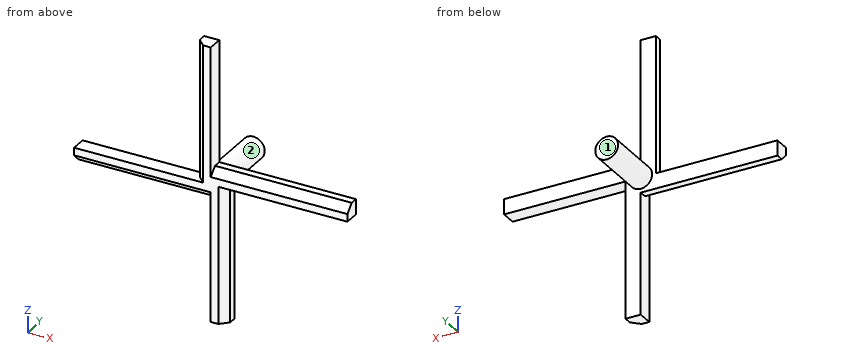
from build123d import *

# Parameters (mm, degrees)
F1_DEPTH = 10
F2_SIZE  = 5
F3_R     = 7.5
F4_DEPTH = 40


with BuildPart() as f1:
    # F0 (on Front) → F1 (new body)
    with BuildSketch(Plane.XZ):
        with BuildLine():
            ThreePointArc((-10, 0), (-7.0710678119, 7.0710678119), (0, 10))
            Line((0, 10), (0, 90))
            Line((0, 90), (-10, 90))
            Line((-10, 90), (-10, 0))
        make_face()
        with BuildLine():
            ThreePointArc((0, -10), (-7.0710678119, -7.0710678119), (-10, 0))
            Line((-10, 0), (-90, 0))
            Line((-90, 0), (-90, -10))
            Line((-90, -10), (0, -10))
        make_face()
        with BuildLine():
            Line((10, -90), (10, 0))
            ThreePointArc((10, 0), (7.0710678119, -7.0710678119), (0, -10))
            Line((0, -10), (0, -90))
            Line((0, -90), (10, -90))
        make_face()
        with BuildLine():
            Line((0, 10), (0, 0))
            Line((0, 0), (10, 0))
            ThreePointArc((10, 0), (7.0710678119, 7.0710678119), (0, 10))
        make_face()
        with BuildLine():
            Line((10, 0), (0, 0))
            Line((0, 0), (0, -10))
            ThreePointArc((0, -10), (7.0710678119, -7.0710678119), (10, 0))
        make_face()
        with BuildLine():
            Line((-10, 0), (0, 0))
            Line((0, 0), (0, 10))
            ThreePointArc((0, 10), (-7.0710678119, 7.0710678119), (-10, 0))
        make_face()
        with BuildLine():
            Line((0, -10), (0, 0))
            Line((0, 0), (-10, 0))
            ThreePointArc((-10, 0), (-7.0710678119, -7.0710678119), (0, -10))
        make_face()
        with BuildLine():
            ThreePointArc((0, 10), (7.0710678119, 7.0710678119), (10, 0))
            Line((10, 0), (90, 0))
            Line((90, 0), (90, 10))
            Line((90, 10), (0, 10))
        make_face()
    extrude(amount=F1_DEPTH)

    # F2
    f2_edges = [f1.edges().sort_by_distance(p)[0] for p in [
        (-10, -10, 45),
        (-45, -10, -10),
        (10, -10, -45),
        (45, -10, 10),
    ]]
    chamfer(f2_edges, length=F2_SIZE)

    # F3 (on Front) → F4 (join)
    with BuildSketch(Plane.XZ):
        Circle(F3_R)
    extrude(amount=-F4_DEPTH)


solid = f1.part
Geometry: final body of the model. Coordinates: model frame, mm. Face numbers are marked on the shaded views. A direction names the side the tool comes from. Give positions to 0.01 mm unless a question says otherwise; leave off trailing zeros. Loops run counter-clockwise (first coordinate to the right, second up) from the corner with the lowest first, then second, coordinate; pieces in that order, holes last. Notation, with made-up numbers: (46, 89.5) -> (101, 89.5) arc R20 cw to (101, 125.5) -> close; hole circle Ø10 at (-38.5, 8.5). An arc over 180 degrees is marked (long way). Put each result on its own line as item: value.
1. Pin query (flat end, axial travel): P1, Ø5.5, axis at x = 52.5, y = -3.5, coming from the +Z side; P2, Ø8, axis at y = -4.5, z = 31.5, coming from the +X side; P3, Ø8, axis at x = -33, y = -7, coming from the +Z side; P4, Ø10, axis at x = -44.5, z = 8, coming from the +Y side. Return the tip coordinate at first contact, or that it passes through.
Taken from the geometry:
P1: stops at z = 10
P2: stops at x = 0
P3: stops at z = 0
P4: passes through
2. Ray query, line 1 along X through (y, z) = (-4.5, 70.5); line 2 along Z through (x, y) = (16.5, -1); line 3 along Z through (x, y) = (6, -1.5). Return the intervals inside material, ascending. Write a range as [from, to].
Taken from the geometry:
line 1: x = [-10, 0]
line 2: z = [0, 10]
line 3: z = [-90, 10]
3. Set-up query: the marked faces 1 and 2. Return all of +Z, -Z, +X, -X, +Y, -Y with unobstructed straight access to the full face (end or side cutting, diameter ignored); none if empty.
Taken from the geometry:
face 1: +Z, -Z, +X, -X, +Y
face 2: +Y
4. Cut plane A-A (z = 21). Return the cut outline in (x, y), plus the area to 3 significant figures.
Taken from the geometry:
outline: (-10, -5) -> (-5, -10) -> (0, -10) -> (0, 0) -> (-10, 0) -> close
area: 87.5 mm2
5. Cut plane C-C (y = 26.5). Return the cut outline in (x, z), plus the area to 3 significant figures.
Taken from the geometry:
outline: circle Ø15 at (0, 0)
area: 177 mm2
